Work out the finished part from the listing and answer in its coordinate system (mm). A direction names the side the tool comes from. Give positions to 0.01 mm unless a question says otherwise; leave off trailing zeros. Loops run counter-clockwise (first coordinate to the right, second up) from the corner with the lowest first, then second, coordinate; pieces in that order, holes last. Notation, with made-up numbers: (62, 58.25) - (101, 58.25) arc R22 ccw to (101, 81.25) - close; hole circle Ø5 at (-29, 51.25). An arc over 180 degrees is marked (long way). Use CSV: the item, a comma, the result in double quotes.
from build123d import *

# Parameters (mm, degrees)
EXTRUDE_1_DEPTH = 5
FILLET_1_R      = 1


with BuildPart() as part:
    # 草圖1 → 填料-伸長1 (new body)
    with BuildSketch(Plane(origin=(0, 0, 0), x_dir=(1, 0, 0), z_dir=(0, 1, 0))):
        Polygon((15, 0), (-15, 0), (-15, 10), (-27, 10), (-27, 23), (-47.5, 58.507041555), (-30.179491924, 68.507041555), (-25.179491924, 59.846787517), (25.179491924, 59.846787517), (30.179491924, 68.507041555), (47.5, 58.507041555), (27, 23), (27, 10), (15, 10), align=None)
    extrude(amount=EXTRUDE_1_DEPTH)

    # 圓角1
    fillet_1_edges = [part.edges().sort_by_distance(p)[0] for p in [
        (-27, 2.5, -10),
        (-27, 2.5, -23),
        (-47.5, 2.5, -58.507041555),
        (-30.179491924, 2.5, -68.507041555),
        (-25.179491924, 2.5, -59.846787517),
        (25.179491924, 2.5, -59.846787517),
        (30.179491924, 2.5, -68.507041555),
        (47.5, 2.5, -58.507041555),
        (27, 2.5, -23),
        (27, 2.5, -10),
        (15, 2.5, -10),
        (15, 2.5, 0),
        (-15, 2.5, 0),
        (-15, 2.5, -10),
    ]]
    fillet(fillet_1_edges, radius=FILLET_1_R)


solid = part.part
Item 1: A cutting plane is placed at B-B on z = -15.5. Determine the outline of the cut face in (x, y).
Determined:
outline,"(-27, 0) - (27, 0) - (27, 5) - (-27, 5) - close"
Item 2: The mould has two halves that part along X. Classify faces 1 (the flat face through (27, 2, -17)), 2 (the flat face through (27.544, 2.465, -63.943)), 3 (the flat face through (1, 5, -35)): pulls with the +X half, pulls with the -X half, needs draft (parallel to the pull), parting line crosses it, or undercut.
Determined:
face 1,"pulls with the +X half"
face 2,"undercut"
face 3,"needs draft"
Item 3: A cutting plane is placed at C-C on x = -22. Determine the outline of the cut face in (y, z).
Determined:
outline,"(0, -59.85) - (5, -59.85) - (5, -10) - (0, -10) - close"
Item 4: For faces 4 (the flat face through (-27.6, 2.46, -64.04)), 5 (the flat face through (15, 2, -5)), 6 (the flat face through (-38.949, 2.465, -63.444)), 7 (the flat face through (-27, 2, -17)), determine the directions among +Z, -Z, +X, -X, +Y, -Y from which every point of the face is accessible in a straight line to the end or side of a thin tool.
Determined:
face 4,"-Z, +Y, -Y"
face 5,"+Z, +X, +Y, -Y"
face 6,"-Z, -X, +Y, -Y"
face 7,"+Z, -X, +Y, -Y"
Item 5: Find the intervals of material crossed by line 1 (Z direction, x = 8, y = 2.75); line 2 (X direction, y = 4.5, z = -18.5); line 3 (X direction, y = 3.6, z = -3.5), in increasing order.
Determined:
line 1,"z = -59.85 to 0"
line 2,"x = -27 to 27"
line 3,"x = -15 to 15"
Item 6: A cutting plane is placed at A-A on y = 3.7. Determine the outline of the cut face in (x, z).
Determined:
outline,"(-47, -57.64) arc R1 ccw to (-46.63, -59.01) - (-31.05, -68.01) arc R1 ccw to (-29.68, -67.64) - (-25.47, -60.35) arc R1 cw to (-24.6, -59.85) - (24.6, -59.85) arc R1 cw to (25.47, -60.35) - (29.68, -67.64) arc R1 ccw to (31.05, -68.01) - (46.63, -59.01) arc R1 ccw to (47, -57.64) - (27.13, -23.23) arc R1 cw to (27, -22.73) - (27, -11) arc R1 ccw to (26, -10) - (16, -10) arc R1 cw to (15, -9) - (15, -1) arc R1 ccw to (14, 0) - (-14, 0) arc R1 ccw to (-15, -1) - (-15, -9) arc R1 cw to (-16, -10) - (-26, -10) arc R1 ccw to (-27, -11) - (-27, -22.73) arc R1 cw to (-27.13, -23.23) - close"
Item 7: Given P1, Ø3, axis at y = 4, z = -7.5, coming from the +X side; P2, Ø1.5, axis at y = 1.5, z = -19.5, coming from the +X side; P3, Ø2, axis at x = 10, y = 3, coming from the -Z side, each flat-ended and moving along its own axis, determine where each tip first touches the part or whether it passes through.
Determined:
P1,"stops at x = 15"
P2,"stops at x = 27"
P3,"stops at z = -59.85"
